The model under review builds one solid part; all positions refer to its coordinate system, in mm. Face numbers are marked on the shaded views. A direction names the side the tool comes from. Coordinates: 2 decimals unless noted, no trailing zeros. Order: outer loops, then holes, each group sorted by start corner. A loop starts at its lowest first (then second) coordinate and runs counter-clockwise, first axis right, second up.
```python
from build123d import *

# Parameters (mm, degrees)
BOSS_EXTRUDE1_DEPTH = 250
SKETCH2_R           = 15
BOSS_EXTRUDE2_DEPTH = 75
BOSS_EXTRUDE3_START = 25
SKETCH3_R           = 15
BOSS_EXTRUDE3_DEPTH = 25
SKETCH4_W           = 12
SKETCH4_H           = 6
CUT_EXTRUDE1_DEPTH  = 50


with BuildPart() as part:
    # Sketch1 → Boss-Extrude1 (new body)
    with BuildSketch(Plane.XY):
        with BuildLine():
            ThreePointArc((0, -20), (19.76835465, -3.035153115), (5.999998319, 19.078784557))
            Line((5.999998319, 19.078784557), (5.999998378, 22.078784557))
            Line((5.999998378, 22.078784557), (0, 22.078784557))
            Line((0, 22.078784557), (0, -20))
        make_face()
        with BuildLine():
            ThreePointArc((-6.000001681, 19.0787835), (-19.768354383, -3.035154857), (0, -20))
            Line((0, -20), (0, 22.078784557))
            Line((0, 22.078784557), (-6.000001622, 22.078784557))
            Line((-6.000001622, 22.078784557), (-6.000001681, 19.0787835))
        make_face()
    extrude(amount=-BOSS_EXTRUDE1_DEPTH)

    # Sketch2 → Boss-Extrude2 (add)
    with BuildSketch(Plane.XY):
        Circle(SKETCH2_R)
    extrude(amount=BOSS_EXTRUDE2_DEPTH)

    # Sketch3 → Boss-Extrude3 (add)
    with BuildSketch(Plane(origin=(0, 0, -250), x_dir=(-1, 0, 0), z_dir=(0, 0, -1)).offset(BOSS_EXTRUDE3_START)):
        with Locations(Location((0, 0, 0), (0, 0, 180))):
            Circle(SKETCH3_R)
    extrude(amount=-BOSS_EXTRUDE3_DEPTH)

    # Sketch4 → Cut-Extrude1 (cut)
    with BuildSketch(Plane.XY.offset(75)):
        with Locations((0, 15)):
            Rectangle(SKETCH4_W, SKETCH4_H)
    extrude(amount=-CUT_EXTRUDE1_DEPTH, mode=Mode.SUBTRACT)


solid = part.part
```
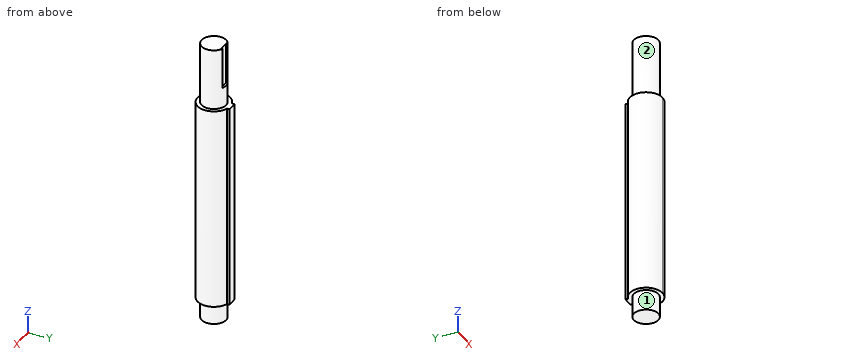
(1) We need section B-B, the plane z = -240.5. Write out the cut boundary in (x, y), and give its area (3 significant figures).
A:
outline: (-6, 19.08) arc R20 ccw (long way) to (6, 19.08) - (6, 22.08) - (-6, 22.08) - close
area: 1,290 mm2
(2) Machinability: for the marked faces 1 and 2, which of the approach directions +Z, -Z, +X, -X, +Y, -Y give a long, thin tool a straight path to every point of the face, cutting with its end or side? Answer none if there is none.
A:
face 1: -Z
face 2: +Z
(3) Wall thickness on probe 1 along Z at (x, y) = (-9, 15); probe 2 along X at (y, z) = (0, -65.5); probe 3 along X at (y, z) = (12, -146): over which ranges is each line inside the solid? List them lowest first.
A:
probe 1: z = -250 to 0
probe 2: x = -20 to 20
probe 3: x = -16 to 16
(4) For pin 1 Ø3.5 at (y, z) = (20, -145.5) entering from -X; pin 2 Ø3 at (y, z) = (8.5, -96.5) entering from +X (3 decimals); pin 3 Ø1.5 at (x, y) = (-1, 13.5) entering from +Z, all flat-tipped, find the tip position at first contact; note any pin that passes through.
A:
pin 1: stops at x = -8.18
pin 2: stops at x = 18.735
pin 3: stops at z = 25
(5) We need section A-A, the plane y = 0. Write out the cut boundary in (x, z), and give its area (3 significant figures).
A:
outline: (-20, -250) - (-15, -250) - (-15, -275) - (15, -275) - (15, -250) - (20, -250) - (20, 0) - (15, 0) - (15, 75) - (-15, 75) - (-15, 0) - (-20, 0) - close
area: 13,000 mm2
